from build123d import *

# Parameters (mm, degrees)
BOSS_EXTRUDE1_DEPTH = 2310
FILLET1_R           = 3
CUT_EXTRUDE1_DEPTH  = 88


with BuildPart() as part:
    # Sketch1 → Boss-Extrude1 (new body)
    with BuildSketch(Plane(origin=(0, 0, 0), x_dir=(0, 0, -1), z_dir=(1, 0, 0))):
        Polygon((0, 0), (85, 0), (85, 82), (47, 82), (47, 112), (50, 112), (50, 85), (88, 85), (88, -3), (0, -3), align=None)
    extrude(amount=BOSS_EXTRUDE1_DEPTH)

    # Fillet1
    fillet1_edges = [part.edges().sort_by_distance(p)[0] for p in [
        (1155, 0, -85),
        (1155, 82, -85),
        (1155, 82, -47),
        (1155, 85, -50),
        (1155, 85, -88),
        (1155, -3, -88),
    ]]
    fillet(fillet1_edges, radius=FILLET1_R)

    # Sketch4 → Cut-Extrude1 (cut)
    with BuildSketch(Plane(origin=(0, 0, -88), x_dir=(-1, 0, 0), z_dir=(0, 0, -1))):
        Polygon((-2310, -3), (-2195, 112), (-2310, 112), align=None)
    extrude(amount=-CUT_EXTRUDE1_DEPTH, mode=Mode.SUBTRACT)


solid = part.part
Verification items for the finished model (mm, model axes). A direction names the side the tool comes from. Round coordinates to 2 decimals unless told otherwise and drop trailing zeros. Loops run counter-clockwise (first coordinate to the right, second up) from the corner with the lowest first, then second, coordinate; pieces in that order, holes last. Notation, with made-up numbers: (-20, 3) - (30, 3) arc R21 ccw to (30, 23) - close; hole circle Ø7 at (18.5, 64). An arc over 180 degrees is marked (long way). Use one line per item in the form item = value.
1. Draft check along Y on faces 1 (the flat face through (1137, 42, -88)), 2 (the flat face through (1137, 0, -40)), 3 (the flat face through (1139, -3, -43)). Enter one of: pulls with the +Y half, pulls with the -Y half, needs draft (parallel to the pull), parting line crosses it, or undercut.
A:
face_1 = needs draft
face_2 = undercut
face_3 = pulls with the -Y half
2. Scan lines: probe 1 along Y at (x, z) = (1710, -67); probe 2 along Z at (x, y) = (356, 75); probe 3 along Z at (x, y) = (1978, 97). Record each from-to range of solid material in increasing order.
A:
probe_1 = -3 to 0, 82 to 85
probe_2 = -88 to -85
probe_3 = -50 to -47
3. Section check C-C on z = -22. Record the cut outline in (x, y), and give its area (3 significant figures).
A:
outline = (0, -3) - (2310, -3) - (2307, 0) - (0, 0) - close
area = 6,930 mm²
4. Section check B-B on y = 56. Record the cut outline in (x, z).
A:
outline = (0, -88) - (2251, -88) - (2251, -85) - (0, -85) - close
5. Gauge pin test, flat ends, axial feed: pin 1 Ø24.5 at (x, z) = (1592.5, -22.5) entering from +Y; pin 2 Ø1.5 at (x, y) = (351, 34) entering from +Z; pin 3 Ø8 at (x, y) = (1649.5, 95.5) entering from +Z; pin 4 Ø6 at (y, z) = (90.5, -71) entering from +X. Record the tip position at first contact, or that the pin passes through.
A:
pin_1 = 0
pin_2 = -85
pin_3 = -47
pin_4 = through
6. Section check A-A on x = 1384.5. Record the cut outline in (y, z), and give its area (3 significant figures).
A:
outline = (-3, -85) arc R3 ccw to (0, -88) - (82, -88) arc R3 ccw to (85, -85) - (85, -53) arc R3 cw to (88, -50) - (112, -50) - (112, -47) - (85, -47) arc R3 ccw to (82, -50) - (82, -82) arc R3 cw to (79, -85) - (3, -85) arc R3 cw to (0, -82) - (0, 0) - (-3, 0) - close
area = 714 mm²
7. Access from +Z, -Z, +X, -X, +Y, -Y to the whole of each face (thin tool, end or side, straight path). Record for faces 4 (the flat face through (0, 38, -87)), 5 (the flat face through (1136, 40, -85)).
A:
face_4 = +Z, -Z, -X, +Y, -Y
face_5 = +Z, +X, -X
